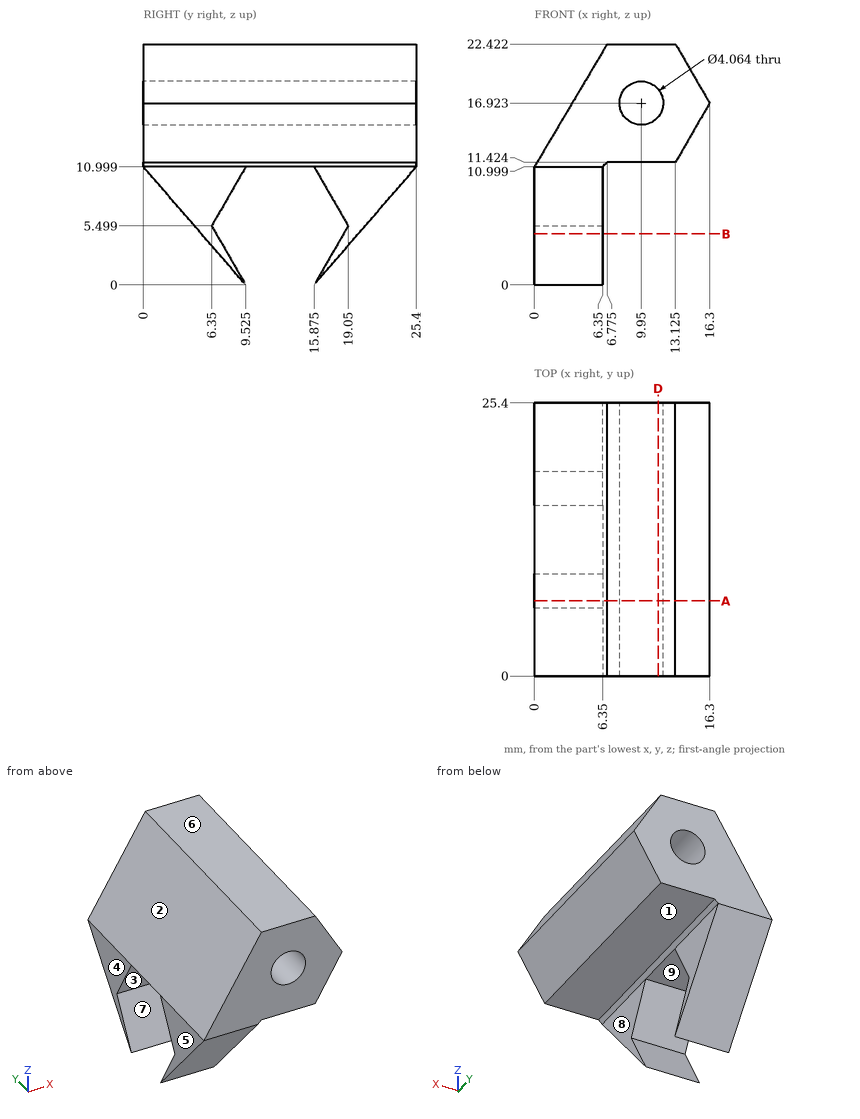
Geometry: see drawing. Coordinates: mm, zero at the bounding-box minimum. A direction names the side the tool comes from. Give positions to 0.01 mm unless a question says otherwise; leave off trailing zeros. Loops run counter-clockwise (first coordinate to the right, second up) from the corner with the lowest first, then second, coordinate; pieces in that order, holes last. Notation, with made-up numbers: (59, 20.25) -> (117, 20.25) arc R16 cw to (117, 47.25) -> close; hole circle Ø4 at (3, 27.25). An arc over 180 degrees is marked (long way). Put each result on its own line as item: value.
1. Set-up query: the marked faces 5, 6, 7, 8 and 9. Return all of +Z, -Z, +X, -X, +Y, -Y with unobstructed straight access to the full face (end or side cutting, diameter ignored); none if empty.
Taken from the geometry:
face 5: +Z, -Z, -X, +Y, -Y
face 6: +Z, +X, -X, +Y, -Y
face 7: +X, -X
face 8: -Z, +X, +Y, -Y
face 9: -Z, +X, -X
2. Cut plane A-A (y = 7). Count the separate pieces of the cut face and the enclosed holes in it, plus the area to 3 significant figures.
Taken from the geometry:
separate pieces: 2
enclosed holes: 1
area: 150 mm2
3. Pull-direction query (Z, two-part tool) for the marked faces 1, 2, 3 and 4; classes: released by +Z, released by -Z, zero draft, split by the parting line, or undercut.
Taken from the geometry:
face 1: released by -Z
face 2: released by +Z
face 3: undercut
face 4: zero draft
4. Cut plane D-D (x = 11.5). Return the cut outline in (y, z).
Taken from the geometry:
outline: (0, 11.42) -> (25.4, 11.42) -> (25.4, 15.61) -> (0, 15.61) -> close; (0, 18.24) -> (25.4, 18.24) -> (25.4, 22.42) -> (0, 22.42) -> close
5. Pin query (flat end, axial travel): P1, Ø12, axis at y = 10.5, z = 14, coming from the +X side; P2, Ø6, axis at x = 2, y = 21.5, coming from the -Z side; P3, Ø10, axis at y = 22, z = 8.5, coming from the +X side (1 decimal). Return the tip coordinate at first contact, or that it passes through.
Taken from the geometry:
P1: stops at x = 16.3
P2: stops at z = 3.03
P3: stops at x = 14.3
6. Cut plane B-B (z = 4.75). Return the cut outline in (x, y).
Taken from the geometry:
outline: (0, 5.41) -> (6.35, 5.41) -> (6.35, 6.78) -> (0, 6.78) -> close; (0, 18.62) -> (6.35, 18.62) -> (6.35, 19.99) -> (0, 19.99) -> close
7. Ray query, line 1 along Z through (x, y) = (10, 1.75) (1 decimal); line 2 along Y through (x, z) = (3.75, 7.5) (1 decimal); line 3 along Z through (x, y) = (10.5, 20.25) (1 decimal). Return the intervals inside material, ascending. Write a range as [from, to].
Taken from the geometry:
line 1: z = [11.4, 14.9], [19, 22.4]
line 2: y = [3, 7.5], [17.9, 22.4]
line 3: z = [11.4, 15], [18.9, 22.4]
